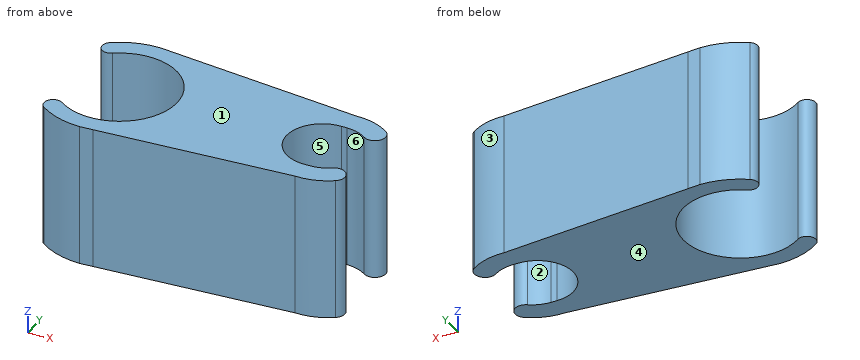
```python
from build123d import *

# Parameters (mm, degrees)
F1_DEPTH = 10


with BuildPart() as f1:
    # F0 (on Top) → F1 (new body)
    with BuildSketch(Plane.XY):
        with BuildLine():
            ThreePointArc((-2.294306, 3.276608), (4, 0), (-2.294306, -3.276608))
            ThreePointArc((-2.294306, -3.276608), (-3.164761, -3.430093), (-3.011276, -4.300548))
            ThreePointArc((-3.011276, -4.300548), (-1.578705, -5.007014), (0, -5.25))
            Line((0, -5.25), (0.901305, -5.172055))
            Line((0.901305, -5.172055), (14.501144, -3.995933))
            ThreePointArc((14.501144, -3.995933), (15.797979, -3.841018), (16.975782, -3.276608))
            ThreePointArc((16.975782, -3.276608), (17.159964, -2.232062), (16.115418, -2.04788))
            ThreePointArc((16.115418, -2.04788), (15.433241, -2.384292), (14.681476, -2.5))
            Line((14.681476, -2.5), (14.281476, -2.5))
            ThreePointArc((14.281476, -2.5), (11.781476, 0), (14.281476, 2.5))
            Line((14.281476, 2.5), (14.681476, 2.5))
            ThreePointArc((14.681476, 2.5), (15.433241, 2.384292), (16.115418, 2.04788))
            ThreePointArc((16.115418, 2.04788), (17.159964, 2.232062), (16.975782, 3.276608))
            ThreePointArc((16.975782, 3.276608), (15.797979, 3.841018), (14.501144, 3.995933))
            Line((14.501144, 3.995933), (0.901305, 5.172055))
            Line((0.901305, 5.172055), (0, 5.25))
            ThreePointArc((0, 5.25), (-1.578705, 5.007014), (-3.011276, 4.300548))
            ThreePointArc((-3.011276, 4.300548), (-3.164761, 3.430093), (-2.294306, 3.276608))
        make_face()
    extrude(amount=F1_DEPTH)


solid = f1.part
```
Work out the finished part from the listing and answer in its coordinate system (mm). Face numbers are marked on the shaded views. A direction names the side the tool comes from. Give positions to 0.01 mm unless a question says otherwise; leave off trailing zeros. Write each loop counter-clockwise with the first axis right and the second up, starting at its lowest first coordinate (ties: lowest second). Pieces come first, ordered by that corner, then holes. Notation, with made-up numbers: (66.25, -36) - (124.25, -36) arc R25 cw to (124.25, -15) - close; hole circle Ø5 at (85, 14.25). An arc over 180 degrees is marked (long way). Use one line per item in the form item = value.
1. Each of these flat-tipped pins is pushed along its axis until it touches: pin 1 Ø1 at (y, z) = (-1, 3) entering from -X; pin 2 Ø1 at (x, y) = (9.5, 1) entering from -Z; pin 3 Ø5 at (x, y) = (0, 0) entering from -Z. Where does it stop, or does it pass through?
Filled in:
pin_1 = 3.71
pin_2 = 0
pin_3 = through
2. Determine the mould class of the marked faces 3, 4, 5 and 6 for opening direction Y: released by +Y, released by -Y, zero draft, split by the parting line, or undercut.
Filled in:
face_3 = released by +Y
face_4 = zero draft
face_5 = undercut
face_6 = undercut
3. A cutting plane is placed at C-C (y = 0). Write down the section's boundary in (x, z), and give its area (3 significant figures).
Filled in:
outline = (4, 0) - (11.78, 0) - (11.78, 10) - (4, 10) - close
area = 77.8 mm^2
4. A cutting plane is placed at A-A (z = 6.25). Write down the section's boundary in (x, y) (3 decimals), and give its area (3 significant figures).
Filled in:
outline = (-3.011, -4.301) arc R5.25 ccw to (0, -5.25) - (0.901, -5.172) - (14.501, -3.996) arc R4 ccw to (16.976, -3.277) arc R0.75 ccw to (16.115, -2.048) arc R2.5 cw to (14.681, -2.5) - (14.281, -2.5) arc R2.5 cw to (14.281, 2.5) - (14.681, 2.5) arc R2.5 cw to (16.115, 2.048) arc R0.75 ccw to (16.976, 3.277) arc R4 ccw to (14.501, 3.996) - (0.901, 5.172) - (0, 5.25) arc R5.25 ccw to (-3.011, 4.301) arc R0.625 ccw to (-2.294, 3.277) arc R4 cw (long way) to (-2.294, -3.277) arc R0.625 ccw to start
area = 115 mm^2
5. A cutting plane is placed at D-D (x = 13.75). Write down the section's boundary in (y, z), and give its area (3 significant figures).
Filled in:
outline = (-4.06, 0) - (-2.44, 0) - (-2.44, 10) - (-4.06, 10) - close; (2.44, 0) - (4.06, 0) - (4.06, 10) - (2.44, 10) - close
area = 32.4 mm^2
6. A cutting plane is placed at B-B (x = 2.25). Write down the section's boundary in (y, z).
Filled in:
outline = (-5.06, 0) - (-3.31, 0) - (-3.31, 10) - (-5.06, 10) - close; (3.31, 0) - (5.06, 0) - (5.06, 10) - (3.31, 10) - close
7. For the marked faces 1 and 2, determine the directions among +Z, -Z, +X, -X, +Y, -Y from which every point of the face is accessible in a straight line to the end or side of a thin tool.
Filled in:
face_1 = +Z, +X, -X, +Y, -Y
face_2 = +Z, -Z
8. Consider L1, parallel to X at y = 0, z = 6.25; L2, parallel to X at y = 2, z = 9.75; L3, parallel to Y at x = -1.75, z = 8. Determine where each line is inside the solid, lowest interval first.
Filled in:
L1 = 4 to 11.78
L2 = 3.46 to 12.78, 16.19 to 16.9
L3 = -4.95 to -3.6, 3.6 to 4.95
